```python
from build123d import *

# Parameters (mm, degrees)
SKETCH_1_R      = 25
EXTRUDE_1_DEPTH = 200
SKETCH_2_R      = 30
EXTRUDE_2_DEPTH = 3
SKETCH_3_R      = 37
EXTRUDE_3_DEPTH = 15
SKETCH_4_R      = 50
EXTRUDE_4_DEPTH = 65
CHAMFER_1_SIZE2 = 7
CHAMFER_1_SIZE  = 10
CHAMFER_2_SIZE2 = 8
CHAMFER_2_SIZE  = 13
EXTRUDE_5_DEPTH = 17.5
EXTRUDE_6_DEPTH = 25
SKETCH_7_R      = 40
EXTRUDE_7_DEPTH = 25
SKETCH_8_R      = 30
EXTRUDE_8_DEPTH = 6
CHAMFER_3_SIZE2 = 10
CHAMFER_3_SIZE  = 8
SKETCH_9_R      = 25
EXTRUDE_9_DEPTH = 150


with BuildPart() as part:
    # 草图1 → 凸台-拉伸1 (new body)
    with BuildSketch(Plane.XY):
        Circle(SKETCH_1_R)
    extrude(amount=-EXTRUDE_1_DEPTH)

    # 草图2 → 凸台-拉伸2 (add)
    with BuildSketch(Plane.XY):
        Circle(SKETCH_2_R)
    extrude(amount=EXTRUDE_2_DEPTH)

    # 草图3 → 凸台-拉伸3 (add)
    with BuildSketch(Plane.XY.offset(3)):
        Circle(SKETCH_3_R)
    extrude(amount=EXTRUDE_3_DEPTH)

    # 草图4 → 凸台-拉伸4 (add)
    with BuildSketch(Plane.XY.offset(18)):
        Circle(SKETCH_4_R)
    extrude(amount=EXTRUDE_4_DEPTH)

    # 倒角1
    chamfer_1_edges = [part.edges().sort_by_distance(p)[0] for p in [
        (-37, 0, 3),
    ]]
    chamfer_1_side = [part.faces().sort_by_distance(p)[0] for p in [
        (-37, 0, 3.14),
    ]]
    chamfer(chamfer_1_edges, length=CHAMFER_1_SIZE - 0.0001, length2=CHAMFER_1_SIZE2 - 0.0001, reference=chamfer_1_side[0])  # a hair under: the kernel refuses the full size

    # 倒角2
    chamfer_2_edges = [part.edges().sort_by_distance(p)[0] for p in [
        (-50, 0, 18),
    ]]
    chamfer_2_side = [part.faces().sort_by_distance(p)[0] for p in [
        (-49.84, 0, 18),
    ]]
    chamfer(chamfer_2_edges, length=CHAMFER_2_SIZE - 0.0001, length2=CHAMFER_2_SIZE2 - 0.0001, reference=chamfer_2_side[0])  # a hair under: the kernel refuses the full size

    # 草图5 → 凸台-拉伸5 (add, symmetric)
    with BuildSketch(Plane.XY.offset(58)):
        with BuildLine():
            Line((-1.99920032, 49.960015994), (-250, 45))
            ThreePointArc((-250, 45), (-295, 0), (-250, -45))
            Line((-250, -45), (-1.99920032, -49.960015994))
            ThreePointArc((-1.99920032, -49.960015994), (-50, 0), (-1.99920032, 49.960015994))
        make_face()
    extrude(amount=EXTRUDE_5_DEPTH, both=True)

    # 草图6 → 凸台-拉伸6 (add, symmetric)
    with BuildSketch(Plane.XY.offset(58)):
        with BuildLine():
            Line((-201.461355602, -12), (0, -12))
            Line((0, -12), (0, 12))
            Line((0, 12), (-201.461355602, 12))
            ThreePointArc((-201.461355602, 12), (-300, 0), (-201.461355602, -12))
        make_face()
    extrude(amount=EXTRUDE_6_DEPTH, both=True)

    # 草图7 → 凸台-拉伸7 (add)
    with BuildSketch(Plane.XY.offset(83)):
        with Locations((-250, 0)):
            Circle(SKETCH_7_R)
    extrude(amount=EXTRUDE_7_DEPTH)

    # 草图8 → 凸台-拉伸8 (add)
    with BuildSketch(Plane.XY.offset(108)):
        with Locations((-250, 0)):
            Circle(SKETCH_8_R)
    extrude(amount=EXTRUDE_8_DEPTH)

    # 倒角3
    chamfer_3_edges = [part.edges().sort_by_distance(p)[0] for p in [
        (-290, 0, 108),
    ]]
    chamfer_3_side = [part.faces().sort_by_distance(p)[0] for p in [
        (-290, 0, 107.84),
    ]]
    chamfer(chamfer_3_edges, length=CHAMFER_3_SIZE - 0.0001, length2=CHAMFER_3_SIZE2 - 0.0001, reference=chamfer_3_side[0])  # a hair under: the kernel refuses the full size

    # 草图9 → 凸台-拉伸9 (add)
    with BuildSketch(Plane.XY.offset(114)):
        with Locations((-250, 0)):
            Circle(SKETCH_9_R)
    extrude(amount=EXTRUDE_9_DEPTH)


solid = part.part
```
Build history of the part. All positions in model axes, mm. A direction names the side the tool comes from. Round coordinates to 2 decimals unless told otherwise and drop trailing zeros. Order: outer loops, then holes, each group sorted by start corner. A loop starts at its lowest first (then second) coordinate and runs counter-clockwise, first axis right, second up. Notation, with made-up numbers: (26.25, 79.5) - (82.25, 79.5) arc R23 cw to (82.25, 106.5) - close; hole circle Ø11 at (-16.5, -39.75). An arc over 180 degrees is marked (long way). Use a Markdown table: item, result.
1) Flat gauge pins, fed straight in: pin 1 Ø8 at (x, z) = (-154.5, 80) entering from +Y; pin 2 Ø3 at (x, y) = (11, 1) entering from +Z; pin 3 Ø1 at (x, y) = (-148, -10) entering from -Z. Where does each tip first touch, or does it go through?
Recorded:
| item | result |
|---|---|
| pin 1 | stops at y = 12 |
| pin 2 | stops at z = 83 |
| pin 3 | stops at z = 33 |
2) Tool access for faces 4 (the face through (-7, 25, 0)), 5 (the face through (-289.96, 1.76, 91.38)), 6 (the face through (-204, 1, 33)): list every direction of +Z, -Z, +X, -X, +Y, -Y with a clear straight run to the whole face (end or side of a thin tool).
Recorded:
| item | result |
|---|---|
| face 4 | -Z |
| face 5 | +Z |
| face 6 | -Z, -X, +Y, -Y |
3) Saw through at B-B on z = 160.5. Write the cut outline in (x, y).
Recorded:
| item | result |
|---|---|
| outline | circle Ø50 at (-250, 0) |
4) Saw through at C-C on x = -146. Write the cut outline in (y, z), and give its area (3 significant figures).
Recorded:
| item | result |
|---|---|
| outline | (-47.08, 40.5) - (-12, 40.5) - (-12, 33) - (12, 33) - (12, 40.5) - (47.08, 40.5) - (47.08, 75.5) - (12, 75.5) - (12, 83) - (-12, 83) - (-12, 75.5) - (-47.08, 75.5) - close |
| area | 3,660 mm² |
5) Pull direction X, two halves, no side cores. Call faces 1 (the face through (-279.97, 1.32, 110.96)), 2 (the face through (47.69, 15.02, 54.1)), 3 (the face through (-89, 1, 83)): pulls with the +X half, pulls with the -X half, needs draft (parallel to the pull), parting line crosses it, or undercut.
Recorded:
| item | result |
|---|---|
| face 1 | parting line crosses it |
| face 2 | undercut |
| face 3 | needs draft |
6) Wall check: L1, parallel to Z at x = -181.5, y = 7; L2, parallel to Z at x = -145, y = -17.5; L3, parallel to X at y = 3, z = -134.5. Give the ranges that are in metal, low to high.
Recorded:
| item | result |
|---|---|
| L1 | z = 33 to 83 |
| L2 | z = 40.5 to 75.5 |
| L3 | x = -24.82 to 24.82 |
